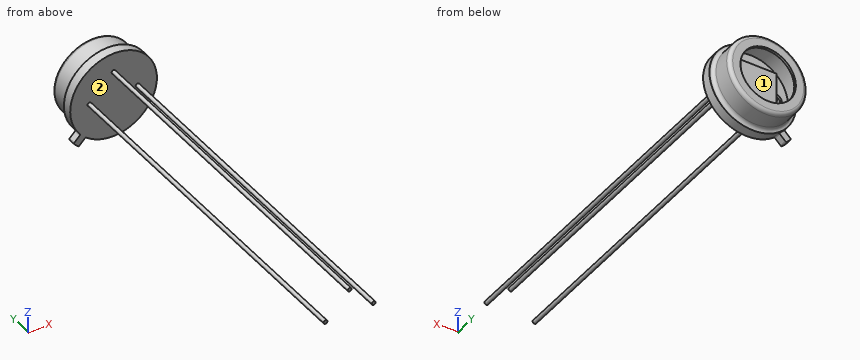
from build123d import *

# Parameters (mm, degrees)
SKETCH1_R                 = 4.1275
BODY_EXTRUDE_DEPTH        = 3.5052
FILLET1_R                 = 0.381
SHELL1_T                  = -0.254
SKETCH2_R                 = 4.572
FLANGE_EXTRUDE_DEPTH      = 1.016
FLANGE_FILLET_R           = 0.381
SKETCH4_R                 = 3.8735
FLANGE_DEPTH_CUTOUT_DEPTH = 0.254
WINDOW_CUTOUT_REACH       = 5.505
SKETCH3_R                 = 2.921
SKETCH6_R                 = 0.6985
PIN_RECESS_DEPTH          = 0.254
SKETCH10_W                = 3.81
SKETCH10_H                = 3.81
BOSS_EXTRUDE1_DEPTH       = 1.1684
SKETCH5_W                 = 3.5999928
SKETCH5_H                 = 3.5999928
DETECTOR_EXTRUDE_DEPTH    = 0.0508
TAB_EXTRUDE_DEPTH         = 0.762
TAB_FILLETS_R             = 0.127
SKETCH8_3_R               = 0.2032
EXTRUDE1_DEPTH            = 38.1
EXTRUDE1_DEPTH_BACK       = 0.762


with BuildPart() as part:
    # Sketch1 → Body Extrude (new body)
    with BuildSketch(Plane(origin=(0, 0, 0), x_dir=(1, 0, 0), z_dir=(0, 1, 0))):
        with Locations(Location((0, 0, 0), (0, 0, 270))):  # turned: the seam where the file's is
            Circle(SKETCH1_R)
    extrude(amount=BODY_EXTRUDE_DEPTH)

    # Fillet1
    fillet1_edges = [part.edges().sort_by_distance(p)[0] for p in [
        (0, 3.5052, -4.1275),
    ]]
    fillet(fillet1_edges, radius=FILLET1_R)

    # Shell1
    shell1_openings = [part.faces().sort_by_distance(p)[0] for p in [
        (0, 0, 0),
    ]]
    offset(amount=SHELL1_T, openings=shell1_openings, kind=Kind.INTERSECTION)

    # Sketch2 → Flange Extrude (add)
    with BuildSketch(Plane(origin=(0, 0, 0), x_dir=(1, 0, 0), z_dir=(0, 1, 0))):
        with Locations(Location((0, 0, 0), (0, 0, 270))):  # turned: the seam where the file's is
            Circle(SKETCH2_R)
    extrude(amount=FLANGE_EXTRUDE_DEPTH)

    # Flange Fillet
    flange_fillet_edges = [part.edges().sort_by_distance(p)[0] for p in [
        (0, 1.016, -4.1275),
    ]]
    fillet(flange_fillet_edges, radius=FLANGE_FILLET_R)

    # Sketch4 → Flange Depth Cutout (cut)
    with BuildSketch(Plane(origin=(0, 1.016, 0), x_dir=(-1, 0, 0), z_dir=(0, 1, 0))):
        with Locations(Location((0, 0, 0), (0, 0, 90))):  # turned: the seam where the file's is
            Circle(SKETCH4_R)
    extrude(amount=-FLANGE_DEPTH_CUTOUT_DEPTH, mode=Mode.SUBTRACT)

    # Sketch3 → Window Cutout (cut, up to next)
    with BuildSketch(Plane(origin=(0, 3.5052, 0), x_dir=(-1, 0, 0), z_dir=(0, 1, 0)), mode=Mode.PRIVATE) as window_cutout_sk1:
        with Locations(Location((0, 0, 0), (0, 0, 90))):  # turned: the seam where the file's is
            Circle(SKETCH3_R)
    window_cutout_tool1 = extrude(window_cutout_sk1.sketch, amount=-WINDOW_CUTOUT_REACH, mode=Mode.PRIVATE) & part.part
    add(window_cutout_tool1.solids().sort_by_distance((0, 3.5052, 0))[0], mode=Mode.SUBTRACT)

    # Sketch6 → Pin Recess (cut)
    with BuildSketch(Plane(origin=(0, 0.762, 0), x_dir=(-1, 0, 0), z_dir=(0, 1, 0))):
        with Locations(Location((-2.54, 0, 0), (0, 0, 90))):  # turned: the seam where the file's is
            Circle(SKETCH6_R)
        with Locations(Location((2.54, 0, 0), (0, 0, 90))):  # turned: the seam where the file's is
            Circle(SKETCH6_R)
    extrude(amount=-PIN_RECESS_DEPTH, mode=Mode.SUBTRACT)

    # Sketch10 → Boss-Extrude1 (add)
    with BuildSketch(Plane(origin=(0, 0.762, 0), x_dir=(1, 0, 0), z_dir=(0, 1, 0))):
        Rectangle(SKETCH10_W, SKETCH10_H)
    extrude(amount=BOSS_EXTRUDE1_DEPTH)

    # Sketch5 → Detector Extrude (add)
    with BuildSketch(Plane(origin=(0, 1.9304, 0), x_dir=(-1, 0, 0), z_dir=(0, 1, 0))):
        Rectangle(SKETCH5_W, SKETCH5_H)
    extrude(amount=DETECTOR_EXTRUDE_DEPTH)

    # Sketch7 → Tab Extrude (add)
    with BuildSketch(Plane(origin=(0, 0, 0), x_dir=(1, 0, 0), z_dir=(0, 1, 0))):
        with BuildLine():
            Line((-3.491055011, 2.952239643), (-4.220720377, 3.68190501))
            Line((-4.220720377, 3.68190501), (-3.68190501, 4.220720377))
            Line((-3.68190501, 4.220720377), (-2.952239643, 3.491055011))
            ThreePointArc((-2.952239643, 3.491055011), (-3.232892204, 3.232892204), (-3.491055011, 2.952239643))
        make_face()
    extrude(amount=TAB_EXTRUDE_DEPTH)

    # Tab Fillets
    tab_fillets_edges = [part.edges().sort_by_distance(p)[0] for p in [
        (-3.491055011, 0.381, -2.952239643),
        (-2.952239643, 0.381, -3.491055011),
        (-3.68190501, 0.381, -4.220720377),
        (-4.220720377, 0.381, -3.68190501),
    ]]
    fillet(tab_fillets_edges, radius=TAB_FILLETS_R)

    # Sketch8_3 → Extrude1 (add, two sides)
    with BuildSketch(Plane.XZ) as extrude1_sk:
        with Locations(Location((2.54, 0, 0), (0, 0, 90))):  # turned: the seam where the file's is
            Circle(SKETCH8_3_R)
        with Locations(Location((0, 2.54, 0), (0, 0, 270))):  # turned: the seam where the file's is
            Circle(SKETCH8_3_R)
        with Locations(Location((-2.54, 0, 0), (0, 0, 90))):  # turned: the seam where the file's is
            Circle(SKETCH8_3_R)
    extrude(amount=EXTRUDE1_DEPTH)
    extrude(extrude1_sk.sketch, amount=-EXTRUDE1_DEPTH_BACK)


solid = part.part
Here's how the part is built. I have some questions about the finished solid (model axes, mm). Face numbers are marked on the shaded views. Round coordinates to 2 decimals unless told otherwise and drop trailing zeros. Loops run counter-clockwise (first coordinate to the right, second up) from the corner with the lowest first, then second, coordinate; pieces in that order, holes last. Notation, with made-up numbers: M 89,4.5 L 106,4.5 A13 ccw 106,25.5 Z; hole C 78.25,-17.75 d6. An arc over 180 degrees is marked long. Write each question's results on one line, items separated by ' | '. Start each with the question number.
(1) Will these pins go through, and if not, where does the flat tip stop? P1, Ø1.5, axis at x = -2, z = 2, coming from the +Y side; P2, Ø1.5, axis at x = -0.5, y = -28.5, coming from the -Z side; P3, Ø2, axis at y = -32.5, z = -0.5, coming from the +X side; P4, Ø1.3, axis at x = -1, y = 1.5, coming from the +Z side.
(2) If I drill on probe 1 along X at (y, z) = (1.8, 0) (1 decimal); probe 2 along Y at (x, z) = (3, -1.5); probe 3 along X at (y, z) = (2.3, 0), over which ranges is the centre line in solid material (lowest first)? Write a range as from..to.
(3) I want a section at A-A (y = -6). Please give me the cut outline in (x, z), then the cut area to 3 significant figures.
(4) Thinking about a two-plate mould opening in Z: for the marked faces 1 and 2, which applies, pulls with the +Z half, pulls with the -Z half, needs draft (parallel to the pull), parting line crosses it, or undercut?
Solved:
1) P1: stops at y = 3.51 | P2: stops at z = 2.34 | P3: stops at x = 2.74 | P4: stops at z = 4.54
2) probe 1: x = -4.1..-3.9, -1.9..1.9, 3.9..4.1 | probe 2: y = 0..0.76, 3.25..3.51 | probe 3: x = -4.13..-3.87, 3.87..4.13
3) outline: C -2.54,0 d0.41; C 0,2.54 d0.41; C 2.54,0 d0.41 | area: 0.389 mm²
4) face 1: undercut | face 2: needs draft
